from build123d import *

# Parameters (mm, degrees)
SKETCH2_W           = 500
SKETCH2_H           = 500
BOSS_EXTRUDE1_DEPTH = 10
CUT_EXTRUDE1_DEPTH  = 5
SKETCH5_W           = 450
SKETCH5_H           = 300
SKETCH5_W_2         = 440
SKETCH5_H_2         = 290
CUT_EXTRUDE2_DEPTH  = 5


with BuildPart() as part:
    # Sketch2 → Boss-Extrude1 (new body)
    with BuildSketch(Plane.XY):
        Rectangle(SKETCH2_W, SKETCH2_H)
    extrude(amount=BOSS_EXTRUDE1_DEPTH)

    # Sketch4 → Cut-Extrude1 (cut)
    with BuildSketch(Plane.XY.offset(10)):
        with BuildLine():
            Line((241.065145693, -229.240987046), (241.219730906, -101.53377405))
            Line((241.219730906, -101.53377405), (-241.170400919, -101.53377405))
            Line((-241.170400919, -101.53377405), (-241.170400919, -228.946326042))
            ThreePointArc((-241.170400919, -228.946326042), (-237.553979354, -238.125325488), (-228.461270123, -241.953533239))
            Line((-228.461270123, -241.953533239), (228.3525995, -241.953533239))
            ThreePointArc((228.3525995, -241.953533239), (237.341727119, -238.230114666), (241.065145693, -229.240987046))
        make_face()
    extrude(amount=-CUT_EXTRUDE1_DEPTH, mode=Mode.SUBTRACT)

    # Sketch5 → Cut-Extrude2 (cut)
    with BuildSketch(Plane.XY.offset(10)):
        with Locations((-8.159820112, 85.603894722)):
            Rectangle(SKETCH5_W, SKETCH5_H)
        with Locations((-8.159820112, 85.603894722)):
            Rectangle(SKETCH5_W_2, SKETCH5_H_2, mode=Mode.SUBTRACT)
    extrude(amount=-CUT_EXTRUDE2_DEPTH, mode=Mode.SUBTRACT)


solid = part.part
The model under review builds one solid part; all positions refer to its coordinate system, in mm. A direction names the side the tool comes from. Round coordinates to 2 decimals unless told otherwise and drop trailing zeros. Loops run counter-clockwise (first coordinate to the right, second up) from the corner with the lowest first, then second, coordinate; pieces in that order, holes last. Notation, with made-up numbers: (37, 63) -> (43, 63) arc R32 ccw to (43, 98) -> close; hole circle Ø10 at (77, 56.25). An arc over 180 degrees is marked (long way). Write item = value, one per line. Start each with the question number.
Item 1: To check wall thickness, follow L1, parallel to X at y = 158.5, z = 5.25; L2, parallel to Y at x = 190.5, z = 7; L3, parallel to Y at x = 216, z = 9.25. State the ranges of each line that lie inside material, in increasing order.
Item 2: Take a section at C-C on y = -157. Give the boundary of the cut face in (x, z), plus the area to 3 significant figures.
Item 3: Insertion check: pin 1 (6 mm diameter, centred on x = -153, y = -161, fed in from -Z). The pin has a flat end and moves straight along its axis. Give the tip position at first contact, or say it passes through.
Item 4: Take a section at B-B on x = 120. Give the boundary of the cut face in (y, z).
Item 5: Take a section at A-A on z = 6.5. Give the boundary of the cut face in (x, y), plus the area to 3 significant figures.
Item 6: Mouldability with a two-part tool opening along Y and no side actions: class faces 3 (the flat face through (17, -73, 10)), 4 (the cylindrical face through (-237.653, -238.023, 7.535)) as released by +Y, released by -Y, zero draft, split by the parting line, or undercut.
Item 7: Take a section at D-D on y = -213. Give the boundary of the cut face in (x, z), plus the area to 3 significant figures.
Item 8: For faces 1 (the cylindrical face through (237.24, -238.33, 7.54)), 2 (the flat face through (-3, 4, 0)), list the 3-axis set-ups (+Z, -Z, +X, -X, +Y, -Y) from which the entire face can be reached by the end or side of a thin tool; tool diameter is ignored.
Result:
q1.L1 = -250 to -233.16, -228.16 to 211.84, 216.84 to 250
q1.L2 = -250 to -241.95, -101.53 to -64.4, -59.4 to 230.6, 235.6 to 250
q1.L3 = -250 to -241.95, -101.53 to -64.4, 235.6 to 250
q2.outline = (-250, 0) -> (250, 0) -> (250, 10) -> (241.15, 10) -> (241.15, 5) -> (-241.17, 5) -> (-241.17, 10) -> (-250, 10) -> close
q2.area = 2,590 mm²
q3.pin_1 = 0
q4.outline = (-250, 0) -> (250, 0) -> (250, 10) -> (235.6, 10) -> (235.6, 5) -> (230.6, 5) -> (230.6, 10) -> (-59.4, 10) -> (-59.4, 5) -> (-64.4, 5) -> (-64.4, 10) -> (-101.53, 10) -> (-101.53, 5) -> (-241.95, 5) -> (-241.95, 10) -> (-250, 10) -> close
q5.outline = (-250, -250) -> (250, -250) -> (250, 250) -> (-250, 250) -> close; (-228.16, -59.4) -> (211.84, -59.4) -> (211.84, 230.6) -> (-228.16, 230.6) -> close; hole (-241.17, -228.95) arc R12.71 ccw to (-228.46, -241.95) -> (228.35, -241.95) arc R12.71 ccw to (241.07, -229.24) -> (241.22, -101.53) -> (-241.17, -101.53) -> close; hole (-233.16, -64.4) -> (216.84, -64.4) -> (216.84, 235.6) -> (-233.16, 235.6) -> close
q5.area = 175,000 mm²
q6.face_3 = zero draft
q6.face_4 = undercut
q7.outline = (-250, 0) -> (250, 0) -> (250, 10) -> (241.08, 10) -> (241.08, 5) -> (-241.17, 5) -> (-241.17, 10) -> (-250, 10) -> close
q7.area = 2,590 mm²
q8.face_1 = +Z
q8.face_2 = -Z, +X, -X, +Y, -Y
